Could you check a few things on this model? Use its own coordinates, in mm. Face numbers are marked on the shaded views. A direction names the side the tool comes from. Round coordinates to 2 decimals unless told otherwise and drop trailing zeros. Loops run counter-clockwise (first coordinate to the right, second up) from the corner with the lowest first, then second, coordinate; pieces in that order, holes last. Notation, with made-up numbers: (59.5, 79.5) -> (82.5, 79.5) arc R24 cw to (82.5, 112.5) -> close; hole circle Ø10 at (7.5, 39.5). An arc over 180 degrees is marked (long way). One line per item, written item: value.
Autodesk Inventor part; units mm, degrees
ref_plane "Work Plane1" through (0, 0, -106) normal (0, 0, 1) x (1, 0, 0)
ref_plane "YZ Plane" through (0, 0, 0) normal (1, 0, 0) x (0, 1, 0)
ref_plane "XZ Plane" through (0, 0, 0) normal (0, 1, 0) x (-1, 0, 0)
sketch "Sketch1" plane through (0, 0, 0) normal (1, 0, 0) x (0, 1, 0)
  circle A0 centre (0, 0) radius 26.5
  line L0 (-26.5, 0) -> (-26.5, -152)
  line L1 (-26.5, -152) -> (26.5, -152)
  line L2 (26.5, -152) -> (26.5, 0)
  dimension "d0" = 53
  dimension "d1" = 152
extrude "Extrusion1" add sketch "Sketch1" along normal mid plane 55
sketch "Sketch2" plane through (0, 0, 0) normal (0, 1, 0) x (-1, 0, 0)
  line L0 (27.5, -152) -> (-27.5, -152)
  circle A0 centre (0, -152) radius 46
  point P0 (0, 0)
  dimension "d4" = 92
extrude "Extrusion2" add sketch "Sketch2" along normal mid plane 53
ref_plane "Work Plane1" through (0, 0, -106) normal (0, 0, 1) x (1, 0, 0)
sketch "Sketch3" plane through (0, 0, -106) normal (0, 0, 1) x (1, 0, 0)
  circle A0 centre (0, 0) radius 10
  dimension "d13" = 20
extrude "Extrusion3" cut sketch "Sketch3" along normal blind 50
properties part number "thigh"
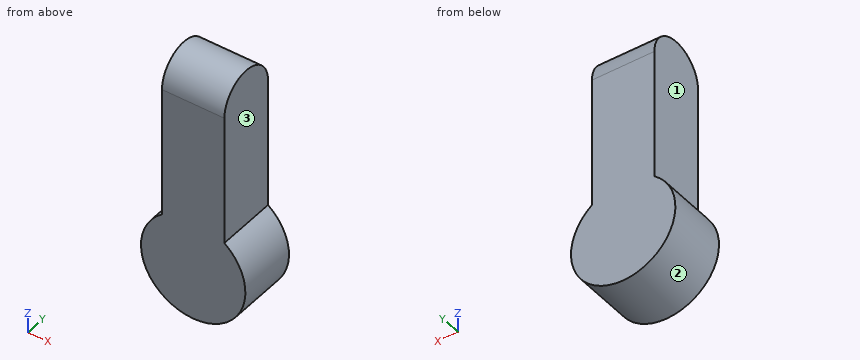
(1) Imagine slicing it at D-D on x = 35. Write out the boundary of the cut face in (y, z), then the cut area to 3 significant figures.
Results below:
outline: (-26.5, -181.85) -> (26.5, -181.85) -> (26.5, -122.15) -> (-26.5, -122.15) -> close
area: 3,160 mm²
(2) Please list where these lines run through material, in increasing order: L1, parallel to Y at x = 0, z = -69; L2, parallel to X at y = -10, z = -50; L3, parallel to Z at x = 34, y = 14.5.
Results below:
L1: y = -26.5 to -10, 10 to 26.5
L2: x = -27.5 to 27.5
L3: z = -182.98 to -121.02
(3) Imagine slicing it at A-A on y = 0. Write out the boundary of the cut face in (x, z), then the cut area to 3 significant figures.
Results below:
outline: (-27.5, -115.13) arc R46 ccw (long way) to (27.5, -115.13) -> (27.5, 26.5) -> (-27.5, 26.5) -> close; hole (-10, -106) -> (10, -106) -> (10, -56) -> (-10, -56) -> close
area: 13,100 mm²
(4) Imagine slicing it at B-B on x = 0. Write out the boundary of the cut face in (y, z).
Results below:
outline: (-26.5, -198) -> (26.5, -198) -> (26.5, 0) arc R26.5 ccw to (-26.5, 0) -> close; hole (-10, -106) -> (10, -106) -> (10, -56) -> (-10, -56) -> close
(5) For pin 1 Ø23 at (x, y) = (0, 0) entering from -Z; pin 2 Ø6 at (y, z) = (-15, -119.5) entering from -X; pin 3 Ø8 at (x, y) = (-28, 0.5) entering from +Z; pin 4 Ø8 at (x, z) = (31, -50.5) entering from -Y, each with a flat end and sliding along its axis, tell me the tip position at first contact or that it passes through.
Results below:
pin 1: stops at z = -198
pin 2: stops at x = -35.3
pin 3: stops at z = 26.5
pin 4: stops at y = -26.5
(6) Imagine slicing it at C-C on z = -49.5. Write out the boundary of the cut face in (x, y), then the cut area to 4 significant figures.
Results below:
outline: (-27.5, -26.5) -> (27.5, -26.5) -> (27.5, 26.5) -> (-27.5, 26.5) -> close
area: 2,915 mm²
(7) On a 3-axis mill with a long thin cutter (end or side, diameter ignored), from which of +Z, -Z, +X, -X, +Y, -Y can I reach the whole of each face in a straight line? I mean the marked faces 1, 2 and 3. Say none if no direction works.
Results below:
face 1: +Z, -X, +Y, -Y
face 2: +Y, -Y
face 3: +Z, +X, +Y, -Y
